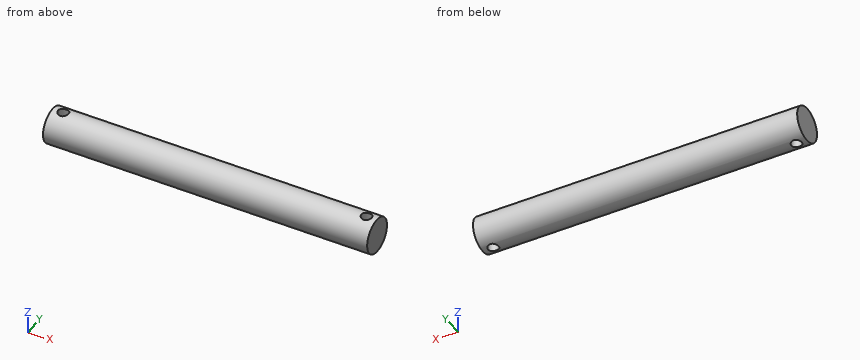
```python
from build123d import *

# Parameters (mm, degrees)
CROQUIS1_R                        = 5
SALIENTE_EXTRUIR1_DEPTH           = 93
CORTAR_EXTRUIR1_REACH             = 7
CROQUIS2_R                        = 1.5
CORTAR_EXTRUIR1_DIRECTION_2_REACH = 7


with BuildPart() as part:
    # Croquis1 → Saliente-Extruir1 (new body)
    with BuildSketch(Plane(origin=(0, 0, 0), x_dir=(0, 0, -1), z_dir=(1, 0, 0))):
        Circle(CROQUIS1_R)
    extrude(amount=SALIENTE_EXTRUIR1_DEPTH)

    # Croquis2 → Cortar-Extruir1 (cut, up to next)
    with BuildSketch(Plane.XY, mode=Mode.PRIVATE) as cortar_extruir1_sk1:
        with Locations((3, 0)):
            Circle(CROQUIS2_R)
    cortar_extruir1_tool1 = extrude(cortar_extruir1_sk1.sketch, amount=-CORTAR_EXTRUIR1_REACH, mode=Mode.PRIVATE) & part.part
    add(cortar_extruir1_tool1.solids().sort_by_distance((3, 0, 0))[0], mode=Mode.SUBTRACT)
    # Croquis2 → Cortar-Extruir1 (cut, up to next)
    with BuildSketch(Plane.XY, mode=Mode.PRIVATE) as cortar_extruir1_sk2:
        with Locations((90, 0)):
            Circle(CROQUIS2_R)
    cortar_extruir1_tool2 = extrude(cortar_extruir1_sk2.sketch, amount=-CORTAR_EXTRUIR1_REACH, mode=Mode.PRIVATE) & part.part
    add(cortar_extruir1_tool2.solids().sort_by_distance((90, 0, 0))[0], mode=Mode.SUBTRACT)

    # Croquis2 → Cortar-Extruir1 direction 2 (cut, up to next)
    with BuildSketch(Plane.XY, mode=Mode.PRIVATE) as cortar_extruir1_direction_2_sk1:
        with Locations((3, 0)):
            Circle(CROQUIS2_R)
    cortar_extruir1_direction_2_tool1 = extrude(cortar_extruir1_direction_2_sk1.sketch, amount=CORTAR_EXTRUIR1_DIRECTION_2_REACH, mode=Mode.PRIVATE) & part.part
    add(cortar_extruir1_direction_2_tool1.solids().sort_by_distance((3, 0, 0))[0], mode=Mode.SUBTRACT)
    # Croquis2 → Cortar-Extruir1 direction 2 (cut, up to next)
    with BuildSketch(Plane.XY, mode=Mode.PRIVATE) as cortar_extruir1_direction_2_sk2:
        with Locations((90, 0)):
            Circle(CROQUIS2_R)
    cortar_extruir1_direction_2_tool2 = extrude(cortar_extruir1_direction_2_sk2.sketch, amount=CORTAR_EXTRUIR1_DIRECTION_2_REACH, mode=Mode.PRIVATE) & part.part
    add(cortar_extruir1_direction_2_tool2.solids().sort_by_distance((90, 0, 0))[0], mode=Mode.SUBTRACT)


solid = part.part
```
Verification items for the finished model (mm, model axes). Round coordinates to 2 decimals unless told otherwise and drop trailing zeros. Order: outer loops, then holes, each group sorted by start corner. A loop starts at its lowest first (then second) coordinate and runs counter-clockwise, first axis right, second up. Notation, with made-up numbers: (-33, 19.25) - (-11, 19.25) arc R24 cw to (-11, 48.25) - close; hole circle Ø8 at (-12.5, 77). An arc over 180 degrees is marked (long way). Use CSV: the item, a comma, the result in double quotes. Start each with the question number.
1) Go/stop test with flat-tipped pins: P1, Ø5, axis at x = 90, y = 0, coming from the +Z side; P2, Ø4, axis at x = 14, y = -3.5, coming from the +Z side; P3, Ø1.5, axis at x = 45, z = -1, coming from the -Y side; P4, Ø2, axis at x = 37, y = -3.5, coming from the -Z side. Record where each tip stops, or that it passes through.
2) Section check C-C, the plane x = 81. Record the cut outline in (y, z), plus the area to 3 significant figures.
3) Thickness scan on L1, parallel to X at y = 0, z = -2.25; L2, parallel to X at y = 0.5, z = -3.75; L3, parallel to Y at x = 90, z = -2. Record the ranges inside material, lowest first.
4) Section check A-A, the plane y = 0. Record the cut outline in (x, z), plus the area to 3 significant figures.
5) Section check D-D, the plane z = -4. Record the cut outline in (x, y), plus the area to 3 significant figures.
6) Section check B-B, the plane z = 0. Record the cut outline in (x, y), plus the area to 3 significant figures.
Answers:
1,P1,"stops at z = 5"
1,P2,"stops at z = 4.77"
1,P3,"stops at y = -4.99"
1,P4,"stops at z = -4.33"
2,outline,"circle Ø10 at (0, 0)"
2,area,"78.5 mm²"
3,L1,"x = 0 to 1.5, 4.5 to 88.5, 91.5 to 93"
3,L2,"x = 0 to 1.59, 4.41 to 88.59, 91.41 to 93"
3,L3,"y = -4.58 to -1.5, 1.5 to 4.58"
4,outline,"(0, -5) - (1.5, -5) - (1.5, 5) - (0, 5) - close; (4.5, -5) - (88.5, -5) - (88.5, 5) - (4.5, 5) - close; (91.5, -5) - (93, -5) - (93, 5) - (91.5, 5) - close"
4,area,"870 mm²"
5,outline,"(0, -3) - (93, -3) - (93, 3) - (0, 3) - close; hole circle Ø3 at (3, 0); hole circle Ø3 at (90, 0)"
5,area,"544 mm²"
6,outline,"(0, -5) - (93, -5) - (93, 5) - (0, 5) - close; hole circle Ø3 at (3, 0); hole circle Ø3 at (90, 0)"
6,area,"916 mm²"
